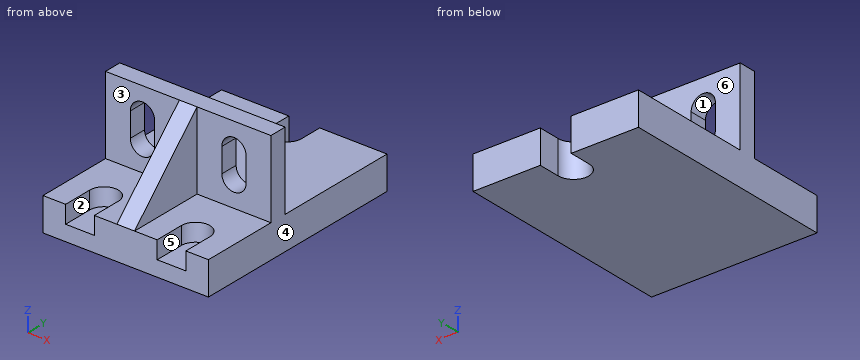
```python
from build123d import *

# Parameters (mm, degrees)
SKETCH_1_W          = 75
SKETCH_1_H          = 100
EXTRUDE_1_DEPTH     = 15
SKETCH_2_W          = 75
SKETCH_2_H          = 8
EXTRUDE_2_DEPTH     = 35
EXTRUDE_3_DEPTH     = 4
CUT_EXTRUDE_1_DEPTH = 91.173443984
CUT_EXTRUDE_2_DEPTH = 8
CUT_EXTRUDE_3_DEPTH = 72.632743909


with BuildPart() as part:
    # Эскиз1 → Бобышка-Вытянуть1 (new body)
    with BuildSketch(Plane.XY):
        Rectangle(SKETCH_1_W, SKETCH_1_H)
    extrude(amount=EXTRUDE_1_DEPTH)

    # Эскиз2 → Бобышка-Вытянуть2 (add)
    with BuildSketch(Plane.XY.offset(15)):
        with Locations((0, -11)):
            Rectangle(SKETCH_2_W, SKETCH_2_H)
    extrude(amount=EXTRUDE_2_DEPTH)

    # Эскиз3 → Бобышка-Вытянуть3 (add, symmetric)
    with BuildSketch(Plane(origin=(0, 0, 0), x_dir=(0, 0, -1), z_dir=(1, 0, 0))):
        Polygon((-50, -15), (-15, -50), (-15, -15), align=None)
    extrude(amount=EXTRUDE_3_DEPTH, both=True)

    # Эскиз4 → Вырез-Вытянуть1 (cut, through all)
    with BuildSketch(Plane.XZ.offset(15)):
        with BuildLine():
            Line((15.25, 27), (15.25, 38))
            ThreePointArc((15.25, 38), (20.75, 43.5), (26.25, 38))
            Line((26.25, 38), (26.25, 27))
            ThreePointArc((26.25, 27), (20.75, 21.5), (15.25, 27))
        make_face()
    cut_extrude_1 = extrude(amount=-CUT_EXTRUDE_1_DEPTH, mode=Mode.SUBTRACT)

    # Эскиз5 → Вырез-Вытянуть2 (cut)
    with BuildSketch(Plane.XY.offset(15)):
        with BuildLine():
            Line((14.25, -63.5), (14.25, -36.5))
            ThreePointArc((14.25, -36.5), (20.75, -30), (27.25, -36.5))
            Line((27.25, -36.5), (27.25, -63.5))
            ThreePointArc((27.25, -63.5), (20.75, -70), (14.25, -63.5))
        make_face()
    cut_extrude_2 = extrude(amount=-CUT_EXTRUDE_2_DEPTH, mode=Mode.SUBTRACT)

    # Эскиз6 → Вырез-Вытянуть3 (cut, through all)
    with BuildSketch(Plane.XY.offset(15)):
        with BuildLine():
            Line((7, 60), (7, 40))
            ThreePointArc((7, 40), (0, 33), (-7, 40))
            Line((-7, 40), (-7, 60))
            ThreePointArc((-7, 60), (0, 67), (7, 60))
        make_face()
    extrude(amount=-CUT_EXTRUDE_3_DEPTH, mode=Mode.SUBTRACT)

    # Зеркальное отражение1: Вырез-Вытянуть1, Вырез-Вытянуть2 across plane
    add(cut_extrude_1.mirror(Plane(origin=(0, 0, 0), x_dir=(0, 0, 1), z_dir=(1, 0, 0))), mode=Mode.SUBTRACT)
    add(cut_extrude_2.mirror(Plane(origin=(0, 0, 0), x_dir=(0, 0, 1), z_dir=(1, 0, 0))), mode=Mode.SUBTRACT)


solid = part.part
```
CAD build for the part. Positions are in the model's coordinates, mm. Face numbers are marked on the shaded views. A direction names the side the tool comes from. Coordinates: 2 decimals unless noted, no trailing zeros. Write each loop counter-clockwise with the first axis right and the second up, starting at its lowest first coordinate (ties: lowest second). Pieces come first, ordered by that corner, then holes. Notation, with made-up numbers: (6, -9.75) -> (49, -9.75) arc R28 cw to (49, 13.25) -> close; hole circle Ø9 at (19.25, 74.25). An arc over 180 degrees is marked (long way). Use CSV: the item, a comma, the result in double quotes. Start each with the question number.
Item 1: Drop flat-ended pins along their axis: P1, Ø4, axis at x = -17.5, y = -39.5, coming from the +Z side; P2, Ø5, axis at x = -15.5, y = -2.5, coming from the +Z side; P3, Ø10.5, axis at y = -37, z = 31.5, coming from the +X side. Give the stop position or say it passes through.
Item 2: Tool access for the marked faces 1, 2 and 3: list every direction of +Z, -Z, +X, -X, +Y, -Y with a clear straight run to the whole face (end or side of a thin tool).
Item 3: Two-plate mould, pull along X, no slides. Class the marked faces 4, 5 and 6: +X half, -X half, draft (parallel to the pull), parting line (faces both ways), or undercut.
Item 4: Band-saw the part on B-B, the plane x = 20.75. Write the cut outline in (y, z).
Item 5: Band-saw the part on D-D, the plane y = -39. Write the cut outline in (x, z).
Item 6: Band-saw the part on C-C, the plane y = 44. Write the cut outline in (x, z).
Item 7: Wall check: probe 1 along X at (y, z) = (-13.5, 35.5); probe 2 along Z at (x, y) = (-6, -29.5); probe 3 along X at (y, z) = (-28.5, 25.5). Give the ranges that are in metal, low to high.
Item 8: Band-saw the part on A-A, the plane z = 34. Write the cut outline in (x, y).
Response values:
1,P1,"stops at z = 7"
1,P2,"stops at z = 15"
1,P3,"stops at x = 4"
2,face 1,"+Y, -Y"
2,face 2,"+Z, -Y"
2,face 3,"+Z, -X, -Y"
3,face 4,"+X half"
3,face 5,"undercut"
3,face 6,"draft"
4,outline,"(-50, 0) -> (50, 0) -> (50, 15) -> (-7, 15) -> (-7, 21.5) -> (-15, 21.5) -> (-15, 15) -> (-30, 15) -> (-30, 7) -> (-50, 7) -> close; (-15, 43.5) -> (-7, 43.5) -> (-7, 50) -> (-15, 50) -> close"
5,outline,"(-37.5, 0) -> (37.5, 0) -> (37.5, 15) -> (27.25, 15) -> (27.25, 7) -> (14.25, 7) -> (14.25, 15) -> (4, 15) -> (4, 26) -> (-4, 26) -> (-4, 15) -> (-14.25, 15) -> (-14.25, 7) -> (-27.25, 7) -> (-27.25, 15) -> (-37.5, 15) -> close"
6,outline,"(-37.5, 0) -> (-7, 0) -> (-7, 15) -> (-37.5, 15) -> close; (7, 0) -> (37.5, 0) -> (37.5, 15) -> (7, 15) -> close"
7,probe 1,"x = -37.5 to -26.25, -15.25 to 15.25, 26.25 to 37.5"
7,probe 2,"z = 0 to 15"
7,probe 3,"x = -4 to 4"
8,outline,"(-37.5, -15) -> (-26.25, -15) -> (-26.25, -7) -> (-37.5, -7) -> close; (-15.25, -15) -> (-4, -15) -> (-4, -31) -> (4, -31) -> (4, -15) -> (15.25, -15) -> (15.25, -7) -> (-15.25, -7) -> close; (26.25, -15) -> (37.5, -15) -> (37.5, -7) -> (26.25, -7) -> close"
